The listing builds one solid part. Answer for the finished solid, in the listing's coordinates (mm). Face numbers are marked on the shaded views. A direction names the side the tool comes from. Round coordinates to 2 decimals unless told otherwise and drop trailing zeros. Write each loop counter-clockwise with the first axis right and the second up, starting at its lowest first coordinate (ties: lowest second). Pieces come first, ordered by that corner, then holes.
(1) The mould has two halves that part along X. Classify the marked faces 1, 2, 3 and 4: +X half, -X half, draft (parallel to the pull), parting line (faces both ways), or undercut.
(2) Each of these flat-tipped pins is pushed along its axis until it touches: pin 1 Ø0.8 at (y, z) = (10.5, 3) entering from +X; pin 2 Ø1.9 at (x, y) = (15, 2.25) entering from -Z; pin 3 Ø1.2 at (x, z) = (13.5, 3.5) entering from -Y; pin 4 Ø3 at (x, z) = (17, 3.5) entering from +Y. Where does it stop, or does it pass through?
(3) A cutting plane is placed at B-B, the plane x = 5. Give the vertices of the cut face in (y, z).
(4) A cutting plane is placed at D-D, the plane y = -0.25. Give the vertices of the cut face in (x, z).
(5) A cutting plane is placed at C-C, the plane z = 3.5. Give the vertices of the cut face in (x, y), and give its area (3 significant figures).
(6) For the marked faces 5, 6, 7 and 8, determine the directions among +Z, -Z, +X, -X, +Y, -Y from which every point of the face is accessible in a straight line to the end or side of a thin tool.
(7) Find the intervals of material crossed by probe 1 along X at (y, z) = (-5.75, 3.5); probe 2 along Y at (x, z) = (15, 2.5); probe 3 along X at (y, z) = (10.25, 2), in increasing order.
(8) A cutting plane is placed at A-A, the plane y = 2.25. Give the vertices of the cut face in (x, z), and give its area (3 significant figures).
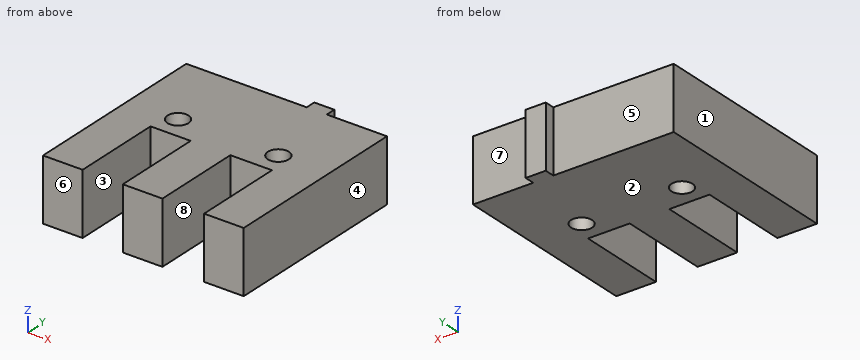
Autodesk Inventor part; units mm, degrees
ref_plane "YZ Plane" through (0, 0, 0) normal (1, 0, 0) x (0, 1, 0)
ref_plane "XZ Plane" through (0, 0, 0) normal (0, 1, 0) x (-1, 0, 0)
ref_plane "XY Plane" through (0, 0, 0) normal (0, 0, 1) x (1, 0, 0)
sketch "Sketch1" plane through (0, 0, 0) normal (0, 0, 1) x (1, 0, 0)
  line L0 (20, 0) -> (20, 10)
  line L1 (20, 10) -> (0, 10)
  line L2 (0, 10) -> (0, 0)
  circle A0 centre (5, 2.25) radius 1.05
  circle A1 centre (15, 2.25) radius 1.05
  line L3 (20, 0) -> (20, -9)
  line L4 (0, -9) -> (0, 0)
  line L5 (3.95, 0) -> (3.95, -9)
  line L6 (16.05, 0) -> (16.05, -9)
  line L7 (7.95, 0) -> (7.95, -9)
  line L8 (7.95, -9) -> (11.9, -9)
  line L9 (11.9, -9) -> (11.9, 0)
  line L10 (3.95, 0) -> (7.95, 0)
  line L11 (11.9, 0) -> (16.05, 0)
  line L12 (3.95, 0) -> (7.95, 0)
  line L13 (11.9, 0) -> (16.05, 0)
  line L14 (3.95, -9) -> (0, -9)
  line L15 (20, -9) -> (16.05, -9)
  line L16 (11.9, -9) -> (7.95, -9)
  line L17 (0, -9) -> (0, 10)
  line L18 (20, 10) -> (0, 10)
  line L19 (20, 10) -> (20, -9)
  line L20 (20, -9) -> (16.05, -9)
  line L21 (16.05, -9) -> (16.05, 0)
  line L22 (16.05, 0) -> (11.9, 0)
  line L23 (11.9, -9) -> (7.95, -9)
  line L24 (7.95, -9) -> (7.95, 0)
  line L25 (7.95, 0) -> (3.95, 0)
  dimension "d0" = 20
  dimension "d1" = 10
  dimension "d2" = 2.1
  dimension "d3" = 2.1
  dimension "d4" = 5
  dimension "d5" = 5
  dimension "d12" = 9
  dimension "d13" = 3.95
  dimension "d14" = 4
extrude "Extrusion3" add sketch "Sketch1" along normal blind 6.2
sketch "Sketch3" plane through (0, 10, 0) normal (0, 1, 0) x (1, 0, 0)
  line L0 (20, 0) -> (0, 0)
  line L1 (20, -6.2) -> (0, -6.2)
  line L2 (20, 0) -> (20, -6.2)
  line L3 (14, 0) -> (14, -6.2)
  line L4 (12, 0) -> (12, -6.2)
  dimension "d17" = 6
  dimension "d18" = 2
extrude "Extrusion4" add sketch "Sketch3" along normal blind 1 contours L3 L1 L4 L0
properties part number "endstop"
Solutions:
1. face 1: -X half
1. face 2: draft
1. face 3: undercut
1. face 4: +X half
2. pin 1: stops at x = 14
2. pin 2: passes through
2. pin 3: stops at y = 0
2. pin 4: stops at y = 10
3. outline: (0, 0) - (1.2, 0) - (1.2, 6.2) - (0, 6.2) - close; (3.3, 0) - (10, 0) - (10, 6.2) - (3.3, 6.2) - close
4. outline: (0, 0) - (3.95, 0) - (3.95, 6.2) - (0, 6.2) - close; (7.95, 0) - (11.9, 0) - (11.9, 6.2) - (7.95, 6.2) - close; (16.05, 0) - (20, 0) - (20, 6.2) - (16.05, 6.2) - close
5. outline: (0, -9) - (3.95, -9) - (3.95, 0) - (7.95, 0) - (7.95, -9) - (11.9, -9) - (11.9, 0) - (16.05, 0) - (16.05, -9) - (20, -9) - (20, 10) - (14, 10) - (14, 11) - (12, 11) - (12, 10) - (0, 10) - close; hole circle Ø2.1 at (5, 2.25); hole circle Ø2.1 at (15, 2.25)
5. area: 302 mm2
6. face 5: +Z, -Z, -X, +Y
6. face 6: +Z, -Z, +X, -X, -Y
6. face 7: +Z, -Z, +X, +Y
6. face 8: +Z, -Z, -Y
7. probe 1: x = 0 to 3.95, 7.95 to 11.9, 16.05 to 20
7. probe 2: y = 0 to 1.2, 3.3 to 10
7. probe 3: x = 12 to 14
8. outline: (0, 0) - (3.95, 0) - (3.95, 6.2) - (0, 6.2) - close; (6.05, 0) - (13.95, 0) - (13.95, 6.2) - (6.05, 6.2) - close; (16.05, 0) - (20, 0) - (20, 6.2) - (16.05, 6.2) - close
8. area: 98.0 mm2
